CAD build for the part. Positions are in the model's coordinates, mm. Face numbers are marked on the shaded views. A direction names the side the tool comes from. Give positions to 0.01 mm unless a question says otherwise; leave off trailing zeros. Loops run counter-clockwise (first coordinate to the right, second up) from the corner with the lowest first, then second, coordinate; pieces in that order, holes last.
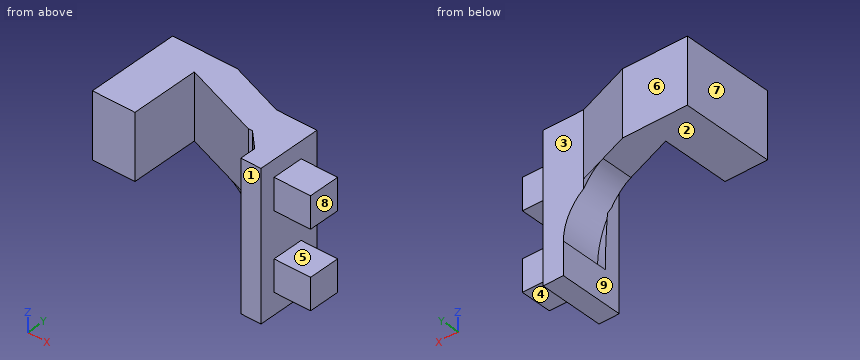
```python
from build123d import *

# Parameters (mm, degrees)
SKETCH1_W           = 5.252522581
SKETCH1_H           = 8.5
BOSS_EXTRUDE1_DEPTH = 4
BOSS_EXTRUDE4_DEPTH = 14
SKETCH1_3_W         = 4.5
SKETCH1_3_H         = 3.875
BOSS_EXTRUDE2_DEPTH = 1.9375
BOSS_EXTRUDE5_START = -11.375
SKETCH1_8_W         = 4.5
SKETCH1_8_H         = 3.875
BOSS_EXTRUDE5_DEPTH = 3.875
FILLET1_R           = 6


with BuildPart() as part:
    # Sketch1 → Boss-Extrude1 (new, symmetric)
    with BuildSketch(Plane.XY):
        Polygon((-5, 7.5), (-4.5, 7.5), (-2.5, 5.5), (-2.5, 3.5), (0, 3.5), (0, 11.5), (-5, 11.5), align=None)
        Polygon((-20, 11.04779164), (-14.747477419, 11.04779164), (-5, 7.5), (-5, 11.5), (-12, 14.04779164), (-20, 14.04779164), align=None)
        with Locations((-17.373738709, 6.79779164)):
            Rectangle(SKETCH1_W, SKETCH1_H)
    extrude(amount=BOSS_EXTRUDE1_DEPTH, both=True)

    # Sketch1<7> → Boss-Extrude4 (add)
    with BuildSketch(Plane.XY):
        Polygon((-2.5, 3.5), (0, 3.5), (0, 5.375), (0, 9.25), (0, 11.5), (-2.5, 11.5), (-2.5, 5.5), align=None)
    extrude(amount=-BOSS_EXTRUDE4_DEPTH)

    # Sketch1<3> → Boss-Extrude2 (add, symmetric)
    with BuildSketch(Plane.XY):
        with Locations((2.25, 7.3125)):
            Rectangle(SKETCH1_3_W, SKETCH1_3_H)
    extrude(amount=BOSS_EXTRUDE2_DEPTH, both=True)

    # Sketch1<8> → Boss-Extrude5 (add)
    with BuildSketch(Plane.XY.offset(BOSS_EXTRUDE5_START)):
        with Locations((2.25, 7.3125)):
            Rectangle(SKETCH1_8_W, SKETCH1_8_H)
    extrude(amount=BOSS_EXTRUDE5_DEPTH)

    # Fillet1
    # the kernel refuses this fillet: 6 mm, written as the material it adds along each edge
    with BuildSketch(Plane(origin=(-2.5, 11.5, -4), x_dir=(-1, 0, 0), z_dir=(0, -1, 0))) as fillet1_piece_1_section:
        with BuildLine():
            CenterArc((FILLET1_R, FILLET1_R), FILLET1_R, 180, 90)
            Line((0, FILLET1_R), (0, 0))
            Line((0, 0), (FILLET1_R, 0))
        make_face()
    fillet1_piece_1 = extrude(amount=21, mode=Mode.PRIVATE)
    fillet1_piece_1 = split(fillet1_piece_1, bisect_by=Plane(origin=(-3.153811187, 10.828042225, -5.911199104), z_dir=(0.3420201433256695, 0.9396926207859081, 0)), keep=Keep.TOP, mode=Mode.PRIVATE)
    add(fillet1_piece_1)
    with BuildSketch(Plane(origin=(-2.5, 26.5, -4), x_dir=(-1, 0, 0), z_dir=(0, -1, 0))) as fillet1_piece_2_section:
        with BuildLine():
            CenterArc((FILLET1_R, FILLET1_R), FILLET1_R, 180, 90)
            Line((0, FILLET1_R), (0, 0))
            Line((0, 0), (FILLET1_R, 0))
        make_face()
    fillet1_piece_2 = extrude(amount=36, mode=Mode.PRIVATE)
    fillet1_piece_2 = split(fillet1_piece_2, bisect_by=Plane(origin=(-6.665111155, 12.106050897, -4.105232665), z_dir=(-0.3420201433256695, -0.9396926207859081, 0)), keep=Keep.TOP, mode=Mode.PRIVATE)
    fillet1_piece_2 = split(fillet1_piece_2, bisect_by=Plane(origin=(-6.768551784, 11.5, -4.105232665), z_dir=(0, 1, 0)), keep=Keep.TOP, mode=Mode.PRIVATE)
    add(fillet1_piece_2)
    with BuildSketch(Plane(origin=(-2.5, 11.5, -4), x_dir=(-1, 0, 0), z_dir=(0, -1, 0))) as fillet1_piece_3_section:
        with BuildLine():
            CenterArc((FILLET1_R, FILLET1_R), FILLET1_R, 180, 90)
            Line((0, FILLET1_R), (0, 0))
            Line((0, 0), (FILLET1_R, 0))
        make_face()
    fillet1_piece_3 = extrude(amount=21, mode=Mode.PRIVATE)
    fillet1_piece_3 = split(fillet1_piece_3, bisect_by=Plane(origin=(-3.734199971, 7.5, -5.388361027), z_dir=(0, 1, 0)), keep=Keep.TOP, mode=Mode.PRIVATE)
    fillet1_piece_3 = split(fillet1_piece_3, bisect_by=Plane(origin=(-3.190866328, 10.841529194, -5.388361027), z_dir=(-0.3420201433256695, -0.9396926207859081, 0)), keep=Keep.TOP, mode=Mode.PRIVATE)
    fillet1_piece_3 = split(fillet1_piece_3, bisect_by=Plane(origin=(-5.041466125, 8.041466125, -5.388361027), z_dir=(0.7071067811865476, 0.7071067811865476, 0)), keep=Keep.TOP, mode=Mode.PRIVATE)
    add(fillet1_piece_3)
    with BuildSketch(Plane(origin=(-2.5, 11.5, -4), x_dir=(-1, 0, 0), z_dir=(0, -1, 0))) as fillet1_piece_4_section:
        with BuildLine():
            CenterArc((FILLET1_R, FILLET1_R), FILLET1_R, 180, 90)
            Line((0, FILLET1_R), (0, 0))
            Line((0, 0), (FILLET1_R, 0))
        make_face()
    fillet1_piece_4 = extrude(amount=21, mode=Mode.PRIVATE)
    fillet1_piece_4 = split(fillet1_piece_4, bisect_by=Plane(origin=(-2.999537912, 7.5, -5.943273976), z_dir=(0, -1, 0)), keep=Keep.TOP, mode=Mode.PRIVATE)
    fillet1_piece_4 = split(fillet1_piece_4, bisect_by=Plane(origin=(-3.116705646, 6.814536913, -5.943273976), z_dir=(0.3420201433256692, 0.9396926207859082, 0)), keep=Keep.TOP, mode=Mode.PRIVATE)
    fillet1_piece_4 = split(fillet1_piece_4, bisect_by=Plane(origin=(-3.567995264, 6.567995264, -5.943273976), z_dir=(0.7071067811865476, 0.7071067811865476, 0)), keep=Keep.TOP, mode=Mode.PRIVATE)
    add(fillet1_piece_4)
    with BuildSketch(Plane(origin=(-2.5, 11.5, -4), x_dir=(-1, 0, 0), z_dir=(0, -1, 0))) as fillet1_piece_5_section:
        with BuildLine():
            CenterArc((FILLET1_R, FILLET1_R), FILLET1_R, 180, 90)
            Line((0, FILLET1_R), (0, 0))
            Line((0, 0), (FILLET1_R, 0))
        make_face()
    fillet1_piece_5 = extrude(amount=21, mode=Mode.PRIVATE)
    fillet1_piece_5 = split(fillet1_piece_5, bisect_by=Plane(origin=(-6.347942504, 7.5, -4.191885591), z_dir=(0, 1, 0)), keep=Keep.TOP, mode=Mode.PRIVATE)
    fillet1_piece_5 = split(fillet1_piece_5, bisect_by=Plane(origin=(-6.566870253, 8.070294133, -4.191885591), z_dir=(0.3420201433256692, 0.9396926207859082, 0)), keep=Keep.TOP, mode=Mode.PRIVATE)
    fillet1_piece_5 = split(fillet1_piece_5, bisect_by=Plane(origin=(-6.009867842, 9.009867842, -4.191885591), z_dir=(-0.7071067811865476, -0.7071067811865476, 0)), keep=Keep.TOP, mode=Mode.PRIVATE)
    add(fillet1_piece_5)
    with BuildSketch(Plane(origin=(-2.5, 11.5, -4), x_dir=(-1, 0, 0), z_dir=(0, -1, 0))) as fillet1_piece_6_section:
        with BuildLine():
            CenterArc((FILLET1_R, FILLET1_R), FILLET1_R, 180, 90)
            Line((0, FILLET1_R), (0, 0))
            Line((0, 0), (FILLET1_R, 0))
        make_face()
    fillet1_piece_6 = extrude(amount=21, mode=Mode.PRIVATE)
    fillet1_piece_6 = split(fillet1_piece_6, bisect_by=Plane(origin=(-2.735586813, 6.675821002, -6.085139246), z_dir=(-0.3420201433256692, -0.9396926207859082, 0)), keep=Keep.TOP, mode=Mode.PRIVATE)
    fillet1_piece_6 = split(fillet1_piece_6, bisect_by=Plane(origin=(-3.085930182, 6.085930182, -6.085139246), z_dir=(0.7071067811865476, 0.7071067811865476, 0)), keep=Keep.TOP, mode=Mode.PRIVATE)
    add(fillet1_piece_6)


solid = part.part
```
1. Drop flat-ended pins along their axis: pin 1 (6 mm diameter, centred on y = 10.5, z = -6.5, fed in from +X); pin 2 (2 mm diameter, centred on x = -0.5, z = -1.5, fed in from -Y); pin 3 (4 mm diameter, centred on y = 8, z = -8.5, fed in from -X); pin 4 (1 mm diameter, centred on x = -14.5, y = 7.5, fed in from -Z). Give the stop position or say it passes through.
Responses:
pin 1: stops at x = 4.5
pin 2: stops at y = 3.5
pin 3: stops at x = -3.63
pin 4: stops at z = -4
2. Probe line 1 along X through (y, z) = (4.5, -9.75); line 2 along Y through (x, z) = (3.25, -7.75) (3 decimals); line 3 along X through (y, z) = (6, -0.5). List the from-to ranges inside material, lowest first.
Responses:
line 1: x = -2.5 to 0
line 2: y = 5.375 to 9.25
line 3: x = -20 to -14.75, -3 to 4.5
3. Saw through at B-B, the plane z = -0.5. List the corners of the cut face in (x, y) (3 decimals).
Responses:
outline: (-20, 2.548) - (-14.747, 2.548) - (-14.747, 11.048) - (-5, 7.5) - (-4.5, 7.5) - (-2.5, 5.5) - (-2.5, 3.5) - (0, 3.5) - (0, 5.375) - (4.5, 5.375) - (4.5, 9.25) - (0, 9.25) - (0, 11.5) - (-5, 11.5) - (-12, 14.048) - (-20, 14.048) - close
4. Pull direction X, two halves, no side cores. Call the marked faces 6, 7, 8 and 9: released by +X, released by -X, zero draft, split by the parting line, or undercut.
Responses:
face 6: zero draft
face 7: released by -X
face 8: released by +X
face 9: undercut
5. Saw through at C-C, the plane y = 8.5. List the corners of the cut face in (x, z) (1 decimal).
Responses:
outline: (-20, -4) - (-14.7, -4) - (-14.7, 4) - (-20, 4) - close; (-7.7, -4) arc R6 cw to (-2.5, -10) - (-2.5, -14) - (0, -14) - (0, -11.4) - (4.5, -11.4) - (4.5, -7.5) - (0, -7.5) - (0, -1.9) - (4.5, -1.9) - (4.5, 1.9) - (0, 1.9) - (0, 4) - (-7.7, 4) - close
6. Tool access for the marked faces 1, 2, 3, 4 and 5: list every direction of +Z, -Z, +X, -X, +Y, -Y with a clear straight run to the whole face (end or side of a thin tool).
Responses:
face 1: +Z, -Z, +X, -Y
face 2: -Z, -X, +Y, -Y
face 3: +Z, -Z, +X, +Y
face 4: -Z, +X, +Y, -Y
face 5: +X, +Y, -Y
7. Saw through at D-D, the plane z = 2.5. List the corners of the cut face in (x, y).
Responses:
outline: (-20, 2.55) - (-14.75, 2.55) - (-14.75, 11.05) - (-5, 7.5) - (-4.5, 7.5) - (-2.5, 5.5) - (-2.5, 3.5) - (0, 3.5) - (0, 11.5) - (-5, 11.5) - (-12, 14.05) - (-20, 14.05) - close
